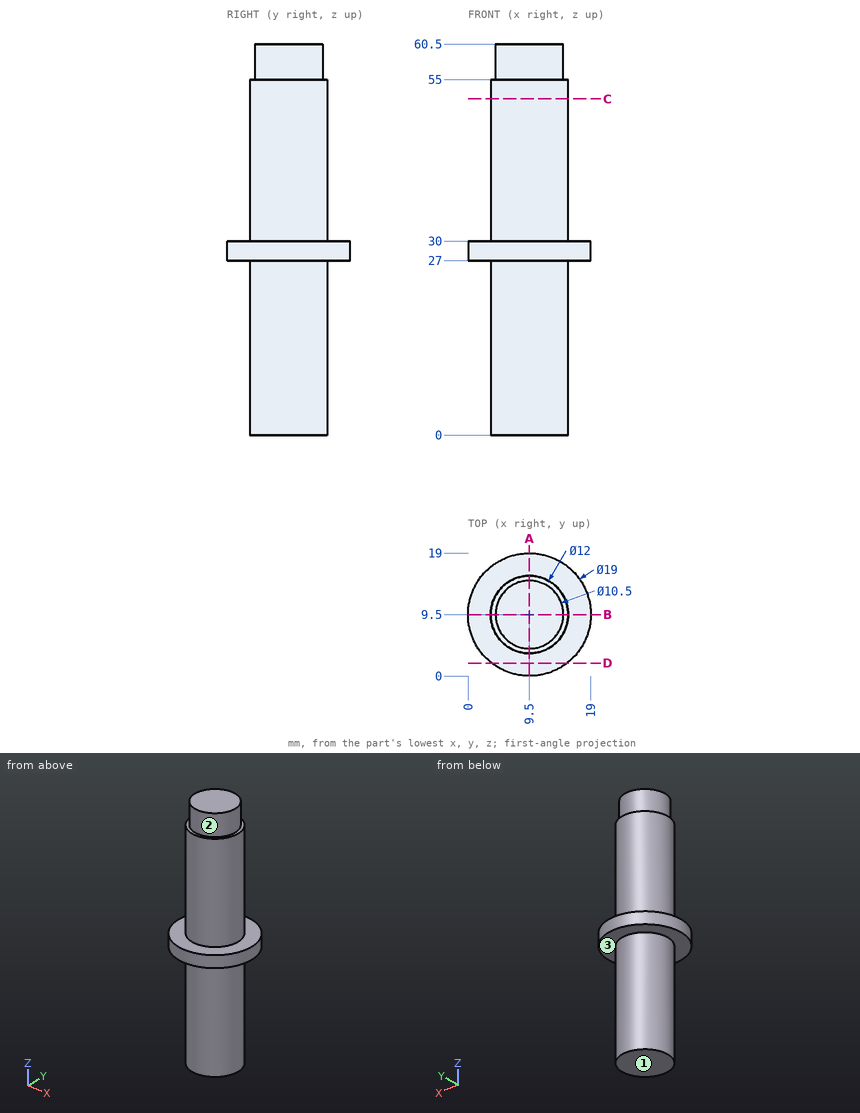
Answer from the drawing. Dimensions are ordinates in mm from the lowest x, y and z of the part. A direction names the side the tool comes from. Coordinates: 2 decimals unless noted, no trailing zeros. Write each loop counter-clockwise with the first axis right and the second up, starting at its lowest first coordinate (ties: lowest second). Pieces come first, ordered by that corner, then holes. Notation, with made-up numbers: M 42,24.5 L 75,24.5 A30 cw 75,61.5 Z; hole C -12,-0.75 d10. An arc over 180 degrees is marked long. Write item = value, one per line.
1. Straight lines are drawn through the part: line 1 (Z direction, x = 2.5, y = 11.25); line 2 (X direction, y = 9.5, z = 45); line 3 (Z direction, x = 7.5, y = 15). For each, find the intervals that lie inside material, in ascending order. Write a range as from..to.
Solution:
line_1 = 27..30
line_2 = 3.5..15.5
line_3 = 0..55
2. The part is cut by section A-A (x = 9.5). Determine the outline of the cut face in (y, z), then the cut area to 3 significant figures.
Solution:
outline = M 0,27 L 3.5,27 L 3.5,0 L 15.5,0 L 15.5,27 L 19,27 L 19,30 L 15.5,30 L 15.5,55 L 14.75,55 L 14.75,60.5 L 4.25,60.5 L 4.25,55 L 3.5,55 L 3.5,30 L 0,30 Z
area = 739 mm2
3. Flat-ended cylindrical pins translate along their axes: pin 1 (5 mm diameter, centred on x = 6.5, z = 16, fed in from +Y); pin 2 (2 mm diameter, centred on x = 12, z = 25.5, fed in from +Y); pin 3 (5 mm diameter, centred on x = 3.5, z = 12.5, fed in from -Y). Find the tip coordinate at first contact, or state that the pin passes through.
Solution:
pin_1 = 15.48
pin_2 = 15.31
pin_3 = 4.63
4. The part is cut by section C-C (z = 52). Determine the outline of the cut face in (x, y).
Solution:
outline = C 9.5,9.5 d12
5. The part is cut by section D-D (y = 2). Determine the outline of the cut face in (x, z), then the cut area to 3 significant figures.
Solution:
outline = M 3.67,27 L 15.33,27 L 15.33,30 L 3.67,30 Z
area = 35.0 mm2
6. For the marked faces 1, 2 and 3, determine the directions among +Z, -Z, +X, -X, +Y, -Y from which every point of the face is accessible in a straight line to the end or side of a thin tool.
Solution:
face_1 = -Z, +X, -X, +Y, -Y
face_2 = +Z
face_3 = -Z
